Geometry: see drawing. Coordinates: mm, zero at the bounding-box minimum. A direction names the side the tool comes from. Give positions to 0.01 mm unless a question says otherwise; leave off trailing zeros. Loops run counter-clockwise (first coordinate to the right, second up) from the corner with the lowest first, then second, coordinate; pieces in that order, holes last. Notation, with made-up numbers: M 52,48 L 92,48 A26 ccw 92,78 Z; hole C 7,-33 d3. An arc over 180 degrees is marked long. Put each result on its own line as item: value.
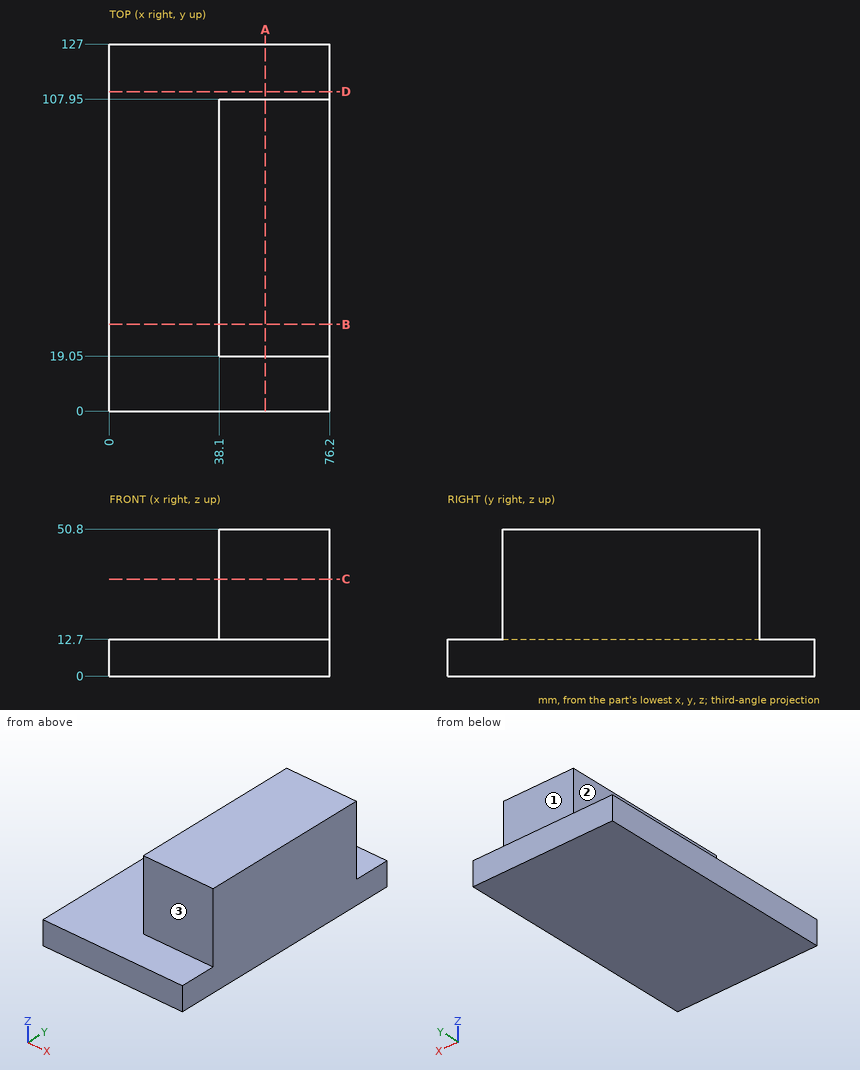
Item 1: Section B-B on y = 30. Output: boundary loops of the cut face in (x, z).
Output values:
outline: M 0,0 L 76.2,0 L 76.2,50.8 L 38.1,50.8 L 38.1,12.7 L 0,12.7 Z
Item 2: Section A-A on x = 54. Output: boundary loops of the cut face in (y, z).
Output values:
outline: M 0,0 L 127,0 L 127,12.7 L 107.95,12.7 L 107.95,50.8 L 19.05,50.8 L 19.05,12.7 L 0,12.7 Z
Item 3: Section C-C on z = 33.5. Output: boundary loops of the cut face in (x, y).
Output values:
outline: M 38.1,19.05 L 76.2,19.05 L 76.2,107.95 L 38.1,107.95 Z
Item 4: Set-up query: the marked faces 1, 2 and 3. Return all of +Z, -Z, +X, -X, +Y, -Y with unobstructed straight access to the full face (end or side cutting, diameter ignored); none if empty.
Output values:
face 1: +Z, +X, -X, +Y
face 2: +Z, -X, +Y, -Y
face 3: +Z, +X, -X, -Y
Item 5: Line query: probe 1 along Z at (x, y) = (11.5, 101.5); probe 2 along Y at (x, z) = (73, 13); probe 3 along X at (y, z) = (56, 45). Output: solid intervals per line, ascending. Write a range as [from, to].
Output values:
probe 1: [0, 12.7]
probe 2: [19.05, 107.95]
probe 3: [38.1, 76.2]
Item 6: Pin query (flat end, axial travel): pin 1 Ø6 at (x, z) = (54.5, 42.5) entering from +Y; pin 2 Ø8 at (x, y) = (29.5, 15.5) entering from +Z. Return the tip coordinate at first contact, or that it passes through.
Output values:
pin 1: y = 107.95
pin 2: z = 12.7
Item 7: Section D-D on y = 110.5. Output: boundary loops of the cut face in (x, z).
Output values:
outline: M 0,0 L 76.2,0 L 76.2,12.7 L 0,12.7 Z
